```python
from build123d import *

# Parameters (mm, degrees)
CHAMFER_1_SIZE      = 0.5
CUT_EXTRUDE_START   = -7
SKETCH_2_R          = 12.139773641
CUT_EXTRUDE_1_DEPTH = 7


with BuildPart() as part:
    # Эскиз1 → Повернуть1 (revolve)
    with BuildSketch(Plane.XY, mode=Mode.PRIVATE) as revolve_1_sk:
        Polygon((0, 47.5), (-5, 47.5), (-5, 17.5), (-9.5, 17.5), (-9.5, 10.5), (-5, 10.5), (-5, 10), (-10, 10), (-50, 5), (-50, 0), (-5, 0), (-5, 7), (0, 7), align=None)
    revolve(revolve_1_sk.sketch.rotate(Axis((0, 0, 0), (0, 1, 0)), 180), axis=Axis((0, 0, 0), (0, 1, 0)))  # turned: the seam where the file's is

    # Фаска1
    chamfer_1_edges = [part.edges().sort_by_distance(p)[0] for p in [
        (-5, 47.5, 0),
    ]]
    chamfer(chamfer_1_edges, length=CHAMFER_1_SIZE)

    # Эскиз2 → Вырез-Вытянуть1 (cut)
    with BuildSketch(Plane(origin=(0, 17.5, 0), x_dir=(1, 0, 0), z_dir=(0, 1, 0)).offset(CUT_EXTRUDE_START)):
        Circle(SKETCH_2_R)
        Polygon((0, 9.5), (-8.227241336, 4.75), (-8.227241336, -4.75), (0, -9.5), (8.227241336, -4.75), (8.227241336, 4.75), align=None, mode=Mode.SUBTRACT)
    extrude(amount=CUT_EXTRUDE_1_DEPTH, mode=Mode.SUBTRACT)


solid = part.part
```
Geometry check sheet. Reference: the model listing, model coordinates, mm. A direction names the side the tool comes from. Coordinates: 2 decimals unless noted, no trailing zeros. Order: outer loops, then holes, each group sorted by start corner. A loop starts at its lowest first (then second) coordinate and runs counter-clockwise, first axis right, second up. Notation, with made-up numbers: (80.25, -25) - (84.25, -25) arc R34 ccw to (84.25, 7) - close; hole circle Ø2 at (84, 4). An arc over 180 degrees is marked (long way). Answer as a JSON object with one key per item and string values. Group by question number.
Item 1: Sectioned sample at A-A, the plane z = 0. Record the cut outline in (x, y), and give its area (3 significant figures).
Item 2: Scan lines: probe 1 along Z at (x, y) = (0, 2); probe 2 along X at (y, z) = (19.5, -1.5); probe 3 along Z at (x, y) = (-4.5, 11.5). Record each from-to range of solid material in increasing order.
Item 3: Depth check by flat-ended pin: pin 1 Ø2 at (x, y) = (-11, 14.5) entering from +Z; pin 2 Ø10 at (y, z) = (8.5, -38) entering from -X; pin 3 Ø3 at (x, z) = (-1, 1.5) entering from -Y; pin 4 Ø1 at (x, z) = (26.5, -27) entering from -Y. Enter the tip coordinate at first touch or a pass-through.
Item 4: Draft check along X on faces 6 (the face through (-4.995, 10.246, -0.22)), 7 (the face through (-4.171, 13.951, 7.092)), 8 (the face through (0, 7, 0)), 9 (the face through (-5, 4, 0)). Enter one of: +X half, -X half, draft (parallel to the pull), parting line (faces both ways), or undercut.
Item 5: Tool access check on faces 1 (the face through (-8.227, 14, 0)), 2 (the face through (4, 10.5, 4)), 3 (the face through (4.171, 13.951, -7.092)), 4 (the face through (-4.056, 13.951, -7.158)), 5 (the face through (4.056, 13.951, 7.158)). Record the directions out of +Z, -Z, +X, -X, +Y, -Y that give a thin tool (end or side, any length) a straight path to the whole face; none if there is none.
Resolved:
{
 "1": {"outline": "(-50, 0) - (-5, 0) - (-5, 7) - (5, 7) - (5, 0) - (50, 0) - (50, 5) - (10, 10) - (5, 10) - (5, 10.5) - (8.23, 10.5) - (8.23, 17.5) - (5, 17.5) - (5, 47) - (4.5, 47.5) - (-4.5, 47.5) - (-5, 47) - (-5, 17.5) - (-8.23, 17.5) - (-8.23, 10.5) - (-5, 10.5) - (-5, 10) - (-10, 10) - (-50, 5) - close", "area": "1,150 mm^2"},
 "2": {"probe 1": "-50 to -5, 5 to 50", "probe 2": "-4.77 to 4.77", "probe 3": "-6.9 to 6.9"},
 "3": {"pin 1": "through", "pin 2": "x = -36.26", "pin 3": "y = 7", "pin 4": "y = 0"},
 "4": {"face 6": "parting line", "face 7": "-X half", "face 8": "undercut", "face 9": "undercut"},
 "5": {"face 1": "+Z, -Z, -X, +Y", "face 2": "none", "face 3": "-Z, +X, +Y", "face 4": "-Z, -X, +Y", "face 5": "+Z, +X, +Y"}
}
